Check sheet for the modelled part. Datum: model origin and axes. Units: mm. A direction names the side the tool comes from. Give positions to 0.01 mm unless a question says otherwise; leave off trailing zeros. Write each loop counter-clockwise with the first axis right and the second up, starting at its lowest first coordinate (ties: lowest second). Pieces come first, ordered by that corner, then holes. Notation, with made-up numbers: M 40.5,-19.5 L 84.5,-19.5 A38 ccw 84.5,18.5 Z; hole C 52.5,84 d5. An arc over 180 degrees is marked long. Write item = value, one per line. Start each with the question number.
1) Cross-section at A-A, the plane z = -1.75. Record the cut outline in (x, y).
2) Cross-section at B-B, the plane x = 12.5. Record the cut outline in (y, z).
3) Scan lines: line 1 along Y through (x, z) = (7.5, 1.5); line 2 along Z through (x, y) = (12.25, -0.5); line 3 along Z through (x, y) = (13.75, 4). Record each from-to range of solid material in increasing order. Write a range as [from, to].
4) Cross-section at C-C, the plane x = 7.75. Record the cut outline in (y, z).
5) Cross-section at D-D, the plane x = 16.5. Record the cut outline in (y, z).
6) Go/stop test with flat-tipped pins: pin 1 (0.6 mm diameter, centred on y = 1, z = -9, fed in from -X); pin 2 (2 mm diameter, centred on y = 0.5, z = 8.5, fed in from +X); pin 3 (1.6 mm diameter, centred on y = -0.5, z = -9.5, fed in from -X). Record where each tip stops, or that it passes through.
7) Mould release check, pull along Y, two halves, no side actions. Record for faces 1 (the cylindrical face through (13, 0, 11)), 2 (the flat face through (13, 6, 0)), 3 (the flat face through (18, 0, 9)): released by +Y, released by -Y, zero draft, split by the parting line, or undercut.
8) Access from +Z, -Z, +X, -X, +Y, -Y to the whole of each face (thin tool, end or side, straight path). Record for faces 4 (the cylindrical face through (7.598, -0.069, -6.567)), 5 (the cylindrical face through (14.567, 0.069, -6.598)), 6 (the flat face through (13, 5, 0)).
```python
from build123d import *

# Parameters (mm, degrees)
FILLET1_R                            = 0.5
BOSS_EXTRUDE6_REACH                  = 29.964
BOSS_EXTRUDE6_END_RADIUS             = 5
BOSS_EXTRUDE6_DIRECTION_2_REACH      = 29.964
BOSS_EXTRUDE6_DIRECTION_2_END_RADIUS = 5


# Read off the part's stored shape, not the designer's step: Mirror2
with BuildPart() as part:
    # Sweep1: sweep along a path in Sketch2path
    with BuildLine(Plane.XY) as sweep1_path:
        Line((0, 0), (25, 0))
    # Sketch3 → Sweep1 (sweep)
    with BuildSketch(Plane(origin=(0, 0, 0), x_dir=(0, 0, -1), z_dir=(1, 0, 0))):
        with BuildLine():
            Line((-5, 6), (5, 6))
            ThreePointArc((5, 6), (11, 0), (5, -6))
            Line((5, -6), (-5, -6))
            ThreePointArc((-5, -6), (-11, 0), (-5, 6))
        make_face()
        with BuildLine():
            Line((-5, 5), (5, 5))
            ThreePointArc((5, 5), (10, 0), (5, -5))
            Line((5, -5), (-5, -5))
            ThreePointArc((-5, -5), (-10, 0), (-5, 5))
        make_face(mode=Mode.SUBTRACT)
    sweep(path=sweep1_path.line)

    # Fillet1
    fillet1_edges = [part.edges().sort_by_distance(p)[0] for p in [
        (0, 0, -10),
        (0, 5, 0),
        (25, 0, -10),
        (0, 0, 10),
        (25, -5, 0),
        (25, 0, 10),
        (25, 5, 0),
        (0, -5, 0),
    ]]
    fillet(fillet1_edges, radius=FILLET1_R)

    # Boss-Extrude6: up to this cylinder (the profile starts inside it)
    boss_extrude6_end = Plane(origin=(16, 0, 5), z_dir=(-1, 0, 0)) * Cylinder(BOSS_EXTRUDE6_END_RADIUS, 70.928, mode=Mode.PRIVATE)
    # Sketch13 → Boss-Extrude6 (add, up to the surface)
    with BuildSketch(Plane(origin=(0, 0, 0), x_dir=(1, 0, 0), z_dir=(0, 1, 0)), mode=Mode.PRIVATE) as boss_extrude6_sk1:
        with BuildLine():
            Line((15.99, -6), (16.01, -6))
            ThreePointArc((16.01, -6), (17.417142495, -6.582857505), (18, -7.99))
            Line((18, -7.99), (18, -10))
            Line((18, -10), (14, -10))
            Line((14, -10), (14, -7.99))
            ThreePointArc((14, -7.99), (14.582857505, -6.582857505), (15.99, -6))
        make_face()
    boss_extrude6_tool1 = extrude(boss_extrude6_sk1.sketch, amount=BOSS_EXTRUDE6_REACH, mode=Mode.PRIVATE) & boss_extrude6_end
    boss_extrude6 = boss_extrude6_tool1.solids().sort_by_distance((16, 0, 8.184882))[0]
    add(boss_extrude6)

    # Boss-Extrude6 direction 2: up to this cylinder (the profile starts inside it)
    boss_extrude6_direction_2_end = Plane(origin=(16, 0, 5), z_dir=(-1, 0, 0)) * Cylinder(BOSS_EXTRUDE6_DIRECTION_2_END_RADIUS, 70.928, mode=Mode.PRIVATE)
    # Sketch13 → Boss-Extrude6 direction 2 (add, up to the surface)
    with BuildSketch(Plane(origin=(0, 0, 0), x_dir=(1, 0, 0), z_dir=(0, 1, 0)), mode=Mode.PRIVATE) as boss_extrude6_direction_2_sk1:
        with BuildLine():
            Line((15.99, -6), (16.01, -6))
            ThreePointArc((16.01, -6), (17.417142495, -6.582857505), (18, -7.99))
            Line((18, -7.99), (18, -10))
            Line((18, -10), (14, -10))
            Line((14, -10), (14, -7.99))
            ThreePointArc((14, -7.99), (14.582857505, -6.582857505), (15.99, -6))
        make_face()
    boss_extrude6_direction_2_tool1 = extrude(boss_extrude6_direction_2_sk1.sketch, amount=-BOSS_EXTRUDE6_DIRECTION_2_REACH, mode=Mode.PRIVATE) & boss_extrude6_direction_2_end
    boss_extrude6_direction_2 = boss_extrude6_direction_2_tool1.solids().sort_by_distance((16, 0, 8.184882))[0]
    add(boss_extrude6_direction_2)
    boss_extrude6 = boss_extrude6 + boss_extrude6_direction_2  # both directions under the feature's name, for the pattern or mirror that repeats it

    # Mirror1: Boss-Extrude6 across plane
    add(boss_extrude6.mirror(Plane(origin=(12.5, 0, 0), x_dir=(0, 0, 1), z_dir=(1, 0, 0))))

    # Mirror2: part across plane


with BuildPart() as part_1:
    add(part.part)
    add(part.part.mirror(Plane.XY))


solid = part_1.part
```
Reply:
q1.outline = M 0,-6 L 25,-6 L 25,-5.5 A0.5 ccw 24.5,-5 L 0.5,-5 A0.5 ccw 0,-5.5 Z; M 0,5.5 A0.5 ccw 0.5,5 L 24.5,5 A0.5 ccw 25,5.5 L 25,6 L 0,6 Z
q2.outline = M -6,-5 A6 ccw 6,-5 L 6,5 A6 ccw -6,5 Z; hole M -5,-5 A5 ccw 5,-5 L 5,5 A5 ccw -5,5 Z
q3.line_1 = [-6, -5], [5, 6]
q3.line_2 = [-10.98, -9.97], [9.97, 10.98]
q3.line_3 = [-9.47, -8], [8, 9.47]
q4.outline = M -6,-5 A6 ccw 6,-5 L 6,5 A6 ccw -6,5 Z; hole M -5,-5 A5 ccw -4.79,-6.43 L 4.79,-6.43 A5 ccw 5,-5 L 5,5 A5 ccw 4.79,6.43 L -4.79,6.43 A5 ccw -5,5 Z
q5.outline = M -6,-5 A6 ccw 6,-5 L 6,5 A6 ccw -6,5 Z; hole M -5,-5 A5 ccw -4.89,-6.06 L 4.89,-6.06 A5 ccw 5,-5 L 5,5 A5 ccw 4.89,6.06 L -4.89,6.06 A5 ccw -5,5 Z
q6.pin_1 = 7
q6.pin_2 = 18
q6.pin_3 = 0.03
q7.face_1 = split by the parting line
q7.face_2 = released by +Y
q7.face_3 = undercut
q8.face_4 = -X
q8.face_5 = none
q8.face_6 = +X, -X
